```python
from build123d import *

# Parameters (mm, degrees)
SKETCH_1_R               = 28
EXTRUDE_1_DEPTH          = 4
SKETCH_2_R               = 12
EXTRUDE_2_DEPTH          = 22
SKETCH_3_R               = 5
CUT_EXTRUDE_1_DEPTH      = 60
SKETCH_4_R               = 1.5
CUT_EXTRUDE_2_DEPTH      = 7
PATTERN_CIRCULAR_1_COUNT = 6
SKETCH_5_R               = 1.5
CUT_EXTRUDE_3_DEPTH      = 15


with BuildPart() as part:
    # Sketch 1 → Extrude 1 (new body)
    with BuildSketch(Plane.XY):
        Circle(SKETCH_1_R)
    extrude(amount=EXTRUDE_1_DEPTH)

    # Sketch 2 → Extrude 2 (add)
    with BuildSketch(Plane.XY.offset(4)):
        Circle(SKETCH_2_R)
    extrude(amount=EXTRUDE_2_DEPTH)

    # Sketch 3 → Cut-Extrude 1 (cut)
    with BuildSketch(Plane.XY.offset(26)):
        Circle(SKETCH_3_R)
    extrude(amount=-CUT_EXTRUDE_1_DEPTH, mode=Mode.SUBTRACT)

    # Sketch 4 → Cut-Extrude 2 (cut)
    with BuildSketch(Plane(origin=(0, 0, 0), x_dir=(-1, 0, 0), z_dir=(0, 0, -1))):
        with Locations((0, 21.265645264)):
            Circle(SKETCH_4_R)
    cut_extrude_2 = extrude(amount=-CUT_EXTRUDE_2_DEPTH, mode=Mode.SUBTRACT)

    # Pattern Circular 1: Cut-Extrude 2 ×6 about axis
    pattern_circular_1_axis = Axis((0, 0, 0), (0, 0, 1))
    for i in range(1, PATTERN_CIRCULAR_1_COUNT):
        add(cut_extrude_2.rotate(pattern_circular_1_axis, i * 360 / PATTERN_CIRCULAR_1_COUNT), mode=Mode.SUBTRACT)

    # Sketch 5 → Cut-Extrude 3 (cut)
    with BuildSketch(Plane(origin=(0, 0, 0), x_dir=(1, 0, 0), z_dir=(0, 1, 0))):
        with Locations((0, -16.223306721)):
            Circle(SKETCH_5_R)
    extrude(amount=-CUT_EXTRUDE_3_DEPTH, mode=Mode.SUBTRACT)


solid = part.part
```
The model under review builds one solid part; all positions refer to its coordinate system, in mm. A direction names the side the tool comes from. Coordinates: 2 decimals unless noted, no trailing zeros. Order: outer loops, then holes, each group sorted by start corner. A loop starts at its lowest first (then second) coordinate and runs counter-clockwise, first axis right, second up. Notation, with made-up numbers: (60.5, -4.5) -> (113.5, -4.5) arc R11 ccw to (113.5, 7.5) -> close; hole circle Ø3 at (59, 64.25). An arc over 180 degrees is marked (long way). Answer in a Markdown table with one row per item. Add a question column.
Item 1: We need section B-B on x = 0. Write out the cut boundary in (y, z), plus the area to 3 significant figures.
Item 2: We need section C-C on x = -9. Write out the cut boundary in (y, z).
Item 3: To check wall thickness, follow probe 1 along Y at (x, z) = (0, 1.35); probe 2 along Z at (x, y) = (-8.5, 16); probe 3 along X at (y, z) = (-6, 15.75). State the ranges of each line that lie inside material, in increasing order.
Item 4: Mouldability with a two-part tool opening along Y and no side actions: class faces 4 (the cylindrical face through (19.8, 11.21, 1.97)), 5 (the flat face through (5.2, 0.2, 26)), 6 (the cylindrical face through (-11.99, 0.53, 14.85)) as +Y half, -Y half, draft (parallel to the pull), parting line (faces both ways), or undercut.
Item 5: Clearance check with flat-ended pins moving along their axes: pin 1 (1.5 mm diameter, centred on y = 4, z = 15.5, fed in from -X); pin 2 (2.5 mm diameter, centred on x = 18.42, y = 10.63, fed in from +Z); pin 3 (10 mm diameter, centred on x = 14.5, z = 16.5, fed in from +Y); pin 4 (8 mm diameter, centred on y = 12, z = 7, fed in from -X). State where each tip first meets the part, or that it passes through.
Item 6: We need section D-D on z = 7.5. Write out the cut boundary in (x, y), plus the area to 3 significant figures.
Item 7: Machinability: for faces 1 (the cylindrical face through (0.325, 19.801, 1.972)), 2 (the flat face through (-13, 0, 4)), 3 (the cylindrical face through (-0.195, -8.332, 14.736)), which of the approach directions +Z, -Z, +X, -X, +Y, -Y give a long, thin tool a straight path to every point of the face, cutting with its end or side? Answer none if there is none.
Item 8: We need section A-A on y = 0. Write out the cut boundary in (x, z).
Final values:
| question | item | result |
|---|---|---|
| 1 | outline | (-28, 0) -> (-22.77, 0) -> (-22.77, 4) -> (-28, 4) -> close; (-19.77, 0) -> (-5, 0) -> (-5, 14.72) -> (-12, 14.72) -> (-12, 4) -> (-19.77, 4) -> close; (-12, 17.72) -> (-5, 17.72) -> (-5, 26) -> (-12, 26) -> close; (5, 0) -> (19.77, 0) -> (19.77, 4) -> (12, 4) -> (12, 26) -> (5, 26) -> close; (22.77, 0) -> (28, 0) -> (28, 4) -> (22.77, 4) -> close |
| 1 | area | 447 mm2 |
| 2 | outline | (-26.51, 0) -> (26.51, 0) -> (26.51, 4) -> (7.94, 4) -> (7.94, 26) -> (-7.94, 26) -> (-7.94, 4) -> (-26.51, 4) -> close |
| 3 | probe 1 | y = -28 to -22.77, -19.77 to -5, 5 to 19.77, 22.77 to 28 |
| 3 | probe 2 | z = 0 to 4 |
| 3 | probe 3 | x = -10.39 to -1.42, 1.42 to 10.39 |
| 4 | face 4 | undercut |
| 4 | face 5 | draft |
| 4 | face 6 | parting line |
| 5 | pin 1 | stops at x = -11.55 |
| 5 | pin 2 | passes through |
| 5 | pin 3 | stops at y = 7.33 |
| 5 | pin 4 | stops at x = -26.39 |
| 6 | outline | circle Ø24 at (0, 0); hole circle Ø10 at (0, 0) |
| 6 | area | 374 mm2 |
| 7 | face 1 | +Z, -Z |
| 7 | face 2 | +Z |
| 7 | face 3 | -Y |
| 8 | outline | (-28, 0) -> (-5, 0) -> (-5, 26) -> (-12, 26) -> (-12, 4) -> (-28, 4) -> close; (5, 0) -> (28, 0) -> (28, 4) -> (12, 4) -> (12, 26) -> (5, 26) -> close |
